CAD build for the part. Positions are in the model's coordinates, mm. Round coordinates to 2 decimals unless told otherwise and drop trailing zeros. Loops run counter-clockwise (first coordinate to the right, second up) from the corner with the lowest first, then second, coordinate; pieces in that order, holes last. Notation, with made-up numbers: M 79,-32 L 98,-32 A14 ccw 98,-18 Z; hole C 36,-15.5 d2. An arc over 180 degrees is marked long. Use a Markdown table: item, result. Add a question column.
(1) Band-saw the part on D-D, the plane x = 16.25. Write the cut outline in (y, z).
(2) Band-saw the part on B-B, the plane x = 13. Write the cut outline in (y, z), and give its area (3 significant figures).
(3) Band-saw the part on A-A, the plane y = 665. Write the cut outline in (x, z), and give its area (3 significant figures).
(4) Two-plate mould, pull along Y, no slides. Class faces 1 (the face through (9.8, 667.4, 0.7)), 2 (the face through (13, 650, 1.5)), 3 (the face through (13, 680, 1)), 4 (the face through (9.8, 637.4, 0.7)): released by +Y, released by -Y, zero draft, split by the parting line, or undercut.
(5) Wall check: L1, parallel to Y at x = 13, z = 0.45; L2, parallel to X at y = 665, z = 0.85; L3, parallel to Y at x = 9.5, z = 1.05. Give the ranges that are in metal, low to high.
(6) Band-saw the part on C-C, the plane z = 0.5. Write the cut outline in (x, y), and give its area (3 significant figures).
Autodesk Inventor part; units mm, degrees
ref_plane "YZ Plane" through (0, 0, 0) normal (1, 0, 0) x (0, 1, 0)
ref_plane "XZ Plane" through (0, 0, 0) normal (0, 1, 0) x (-1, 0, 0)
ref_plane "XY Plane" through (0, 0, 0) normal (0, 0, 1) x (1, 0, 0)
sketch "Sketch1" plane through (0, 0, 0) normal (0, 0, 1) x (1, 0, 0)
  arc A0 (11.6513, 631.9608) -> (14.3394, 631.9567) centre (13, 635) ccw
  arc A1 (14.3394, 638.0433) -> (11.6606, 638.0433) centre (13, 635) ccw
  arc A2 (11.6513, 661.9608) -> (14.3394, 661.9567) centre (13, 665) ccw
  arc A3 (14.3394, 668.0433) -> (11.6606, 668.0433) centre (13, 665) ccw
  line L0 (25.9999, 620.0001) -> (17.4375, 620.0001)
  line L1 (0, 679.9999) -> (8.4375, 679.9999)
  circle A4 centre (13, 635) radius 4
  circle A5 centre (13, 665) radius 4
  line L2 (28, 620.0001) -> (-2, 620.0001)
  line L3 (-2, 620.0001) -> (-2, 679.9999)
  line L4 (-2, 679.9999) -> (28, 679.9999)
  line L5 (28, 679.9999) -> (28, 620.0001)
  line L6 (13, 620.0001) -> (13, 679.9999) construction
  point P0 (0, 0)
  dimension "d0" = 8
  dimension "d2" = 30
extrude "Plate1" add sketch "Sketch1" along normal blind 1.5
equation "\"BendRadius\" = Thickness"
equation "\"BendReliefWidth\" = Thickness"
equation "\"BendReliefDepth\" = 0.5 * Thickness"
equation "\"CornerReliefSize\" = 4 * Thickness"
equation "\"MinimumRemnant\" = 2 * Thickness"
equation "\"TransitionRadius\" = BendRadius"
equation "\"JacobiRadiusSize\" = BendRadius"
equation "\"GapSize\" = Thickness"
equation "\"d3\" = BendRadius"
properties part number "gabarito-travessa-60" material "Wood (Oak)"
Return value:
| question | item | result |
|---|---|---|
| 1 | outline | M 620,0 L 632.67,0 L 632.67,1.5 L 620,1.5 Z; M 637.33,0 L 662.67,0 L 662.67,1.5 L 637.33,1.5 Z; M 667.33,0 L 680,0 L 680,1.5 L 667.33,1.5 Z |
| 2 | outline | M 620,0 L 631,0 L 631,1.5 L 620,1.5 Z; M 639,0 L 661,0 L 661,1.5 L 639,1.5 Z; M 669,0 L 680,0 L 680,1.5 L 669,1.5 Z |
| 2 | area | 66.0 mm^2 |
| 3 | outline | M -2,0 L 9,0 L 9,1.5 L -2,1.5 Z; M 17,0 L 28,0 L 28,1.5 L 17,1.5 Z |
| 3 | area | 33.0 mm^2 |
| 4 | face 1 | undercut |
| 4 | face 2 | zero draft |
| 4 | face 3 | released by +Y |
| 4 | face 4 | undercut |
| 5 | L1 | 620 to 631, 639 to 661, 669 to 680 |
| 5 | L2 | -2 to 9, 17 to 28 |
| 5 | L3 | 620 to 633.06, 636.94 to 663.06, 666.94 to 680 |
| 6 | outline | M -2,620 L 28,620 L 28,680 L -2,680 Z; hole C 13,635 d8; hole C 13,665 d8 |
| 6 | area | 1,700 mm^2 |
